The listing builds one solid part. Answer for the finished solid, in the listing's coordinates (mm). Face numbers are marked on the shaded views. A direction names the side the tool comes from. Give positions to 0.01 mm unless a question says otherwise; leave off trailing zeros. Loops run counter-clockwise (first coordinate to the right, second up) from the corner with the lowest first, then second, coordinate; pieces in that order, holes last.
Item 1: Each of these flat-tipped pins is pushed along its axis until it touches: pin 1 Ø10 at (x, z) = (-3, -3.5) entering from +Y; pin 2 Ø6.5 at (x, z) = (0, 20) entering from -Y; pin 3 Ø2 at (y, z) = (12, 23.5) entering from +X; pin 4 Ø10.5 at (x, z) = (-20, -20) entering from -Y. Where does it stop, or does it pass through?
Item 2: Section C-C, the plane x = 0 is taken. Give the vertices of the cut face in (y, z).
Item 3: The mould has two halves that part along Z. Classify the marked faces 1, 2 and 3: pulls with the +Z half, pulls with the -Z half, needs draft (parallel to the pull), parting line crosses it, or undercut.
Item 4: Section A-A, the plane x = 20 is taken. Give the vertices of the cut face in (y, z), and give its area (3 significant figures).
Item 5: Section D-D, the plane z = 0 is taken. Give the vertices of the cut face in (x, y), and give its area (3 significant figures).
Item 6: Consider line 1 along Y through (x, z) = (29, -27); line 2 along X through (y, z) = (3, -20); line 3 along Z through (x, y) = (27, -12). Determine where each line is inside the solid, lowest interval first.
Item 7: A tool of negligible diameter and unlimited length cuts with its end or side. For the marked faces 4 and 5, from which of +Z, -Z, +X, -X, +Y, -Y can it reach the whole face along a straight path? Write none if from no direction.
Item 8: Section B-B, the plane y = 3 is taken. Give the vertices of the cut face in (x, z).
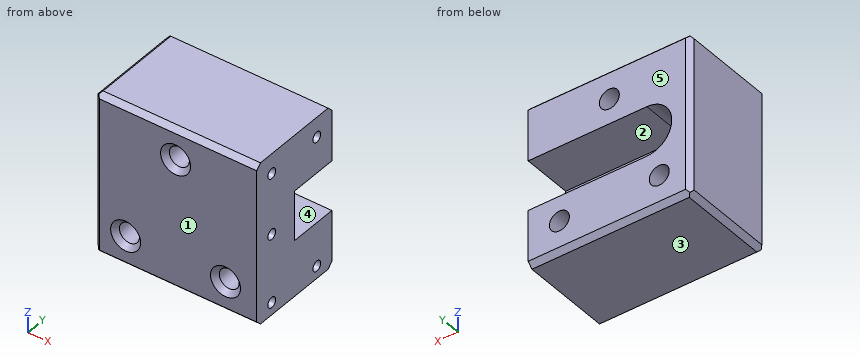
Solid Edge part; units mm, degrees
sketch "Sketch1" plane through (0, 0, 0) normal (0, -1, 0) x (1, 0, 0)
  line L0 (-32.5, 32.5) -> (32.5, 32.5)
  line L1 (32.5, 32.5) -> (32.5, -32.5)
  line L2 (32.5, -32.5) -> (-32.5, -32.5)
  line L3 (-32.5, -32.5) -> (-32.5, 32.5)
  dimension "D1" = 32.5
  dimension "D2" = 32.5
extrude "Protrusion1" add sketch "Sketch1" along normal mid plane 40
hole "Bohrung_1" at (-20, -20, -20) direction (0, 1, 0) diameter 8 end up to next
hole "Hole1" at (20, -20, -20) direction (0, 1, 0) diameter 8 end up to next
hole "Hole2" at (0, -20, 20) direction (0, 1, 0) diameter 8 end up to next
chamfer "Fase_1" distance 2 angle 45 3 edges at (16, -20, -20) (-24, -20, -20) (-4, -20, 20)
chamfer "Fase_2" distance 2 angle 45 3 edges at (0, -20, -32.5) (-32.5, -20, 0) (0, -20, 32.5)
chamfer "Fase_3" distance 2 angle 45 2 edges at (-32.5, 1, -32.5) (-32.5, 1, 32.5)
hole "Bohrung_6" at (-15, 20, 0) direction (0, -1, 0) diameter 20 depth 20
sketch "Sketch2" plane through (0, 20, 0) normal (0, 1, 0) x (1, 0, 0)
  line L0 (-15, 10) -> (32.5, 10)
  line L1 (32.5, 10) -> (32.5, -10)
  line L2 (-15, -10) -> (32.5, -10)
  line L3 (-15, 10) -> (-15, -10)
extrude "Ausschnitt_2" cut sketch "Sketch2" against normal blind 20
hole "Bohrung_7" at (32.5, 12, 24.5) direction (-1, 0, 0) diameter 4.134 depth 25
hole "Hole3" at (32.5, -12, 24.5) direction (-1, 0, 0) diameter 4.134 depth 25
hole "Bohrung_9" at (32.5, -12, 0) direction (-1, 0, 0) diameter 4.134 depth 15
hole "Bohrung_10" at (32.5, 12, -27.5) direction (-1, 0, 0) diameter 4.134 depth 15
hole "Hole4" at (32.5, -12, -27.5) direction (-1, 0, 0) diameter 4.134 depth 15
chamfer "Fase_4" distance 2 angle 45 3 edges at (1, 20, 32.5) (-32.5, 20, 0) (1, 20, -32.5)
properties material "polyamid"
Worked answers:
1. pin 1: stops at y = 0
1. pin 2: passes through
1. pin 3: stops at x = 7.5
1. pin 4: stops at y = -19.25
2. outline: (-20, -30.5) - (-18, -32.5) - (18, -32.5) - (20, -30.5) - (20, -10) - (0, -10) - (0, 10) - (20, 10) - (20, 16) - (-18, 16) - (-20, 14) - close; (-20, 26) - (-18, 24) - (20, 24) - (20, 30.5) - (18, 32.5) - (-18, 32.5) - (-20, 30.5) - close
3. face 1: needs draft
3. face 2: undercut
3. face 3: pulls with the -Z half
4. outline: (-20, -30.5) - (-18, -32.5) - (18, -32.5) - (20, -30.5) - (20, -24) - (-18, -24) - (-20, -26) - close; (-20, -14) - (-18, -16) - (20, -16) - (20, -10) - (0, -10) - (0, 10) - (20, 10) - (20, 30.5) - (18, 32.5) - (-18, 32.5) - (-20, 30.5) - close; hole circle Ø4.13 at (-12, -27.5); hole circle Ø4.13 at (-12, 0); hole circle Ø4.13 at (-12, 24.5); hole circle Ø4.13 at (12, -27.5); hole circle Ø4.13 at (12, 24.5)
4. area: 1,800 mm2
5. outline: (-32.5, -18) - (-30.5, -20) - (32.5, -20) - (32.5, -14.07) - (17.5, -14.07) - (17.5, -9.93) - (32.5, -9.93) - (32.5, 0) - (-25, 0) - (-25, 20) - (-30.5, 20) - (-32.5, 18) - close
5. area: 1,380 mm2
6. line 1: y = -20 to -14.01, -9.99 to 9.99, 14.01 to 20
6. line 2: x = -32.5 to -24, -16 to 16, 24 to 32.5
6. line 3: z = -32.5 to -29.57, -25.43 to -2.07, 2.07 to 22.43, 26.57 to 32.5
7. face 4: +X, +Y
7. face 5: +Z, -Z, +X, -X, +Y
8. outline: (-32.5, -30.5) - (-30.5, -32.5) - (32.5, -32.5) - (32.5, -10) - (-15, -10) arc R10 cw to (-15, 10) - (32.5, 10) - (32.5, 32.5) - (-30.5, 32.5) - (-32.5, 30.5) - close; hole circle Ø8 at (-20, -20); hole circle Ø8 at (0, 20); hole circle Ø8 at (20, -20)
